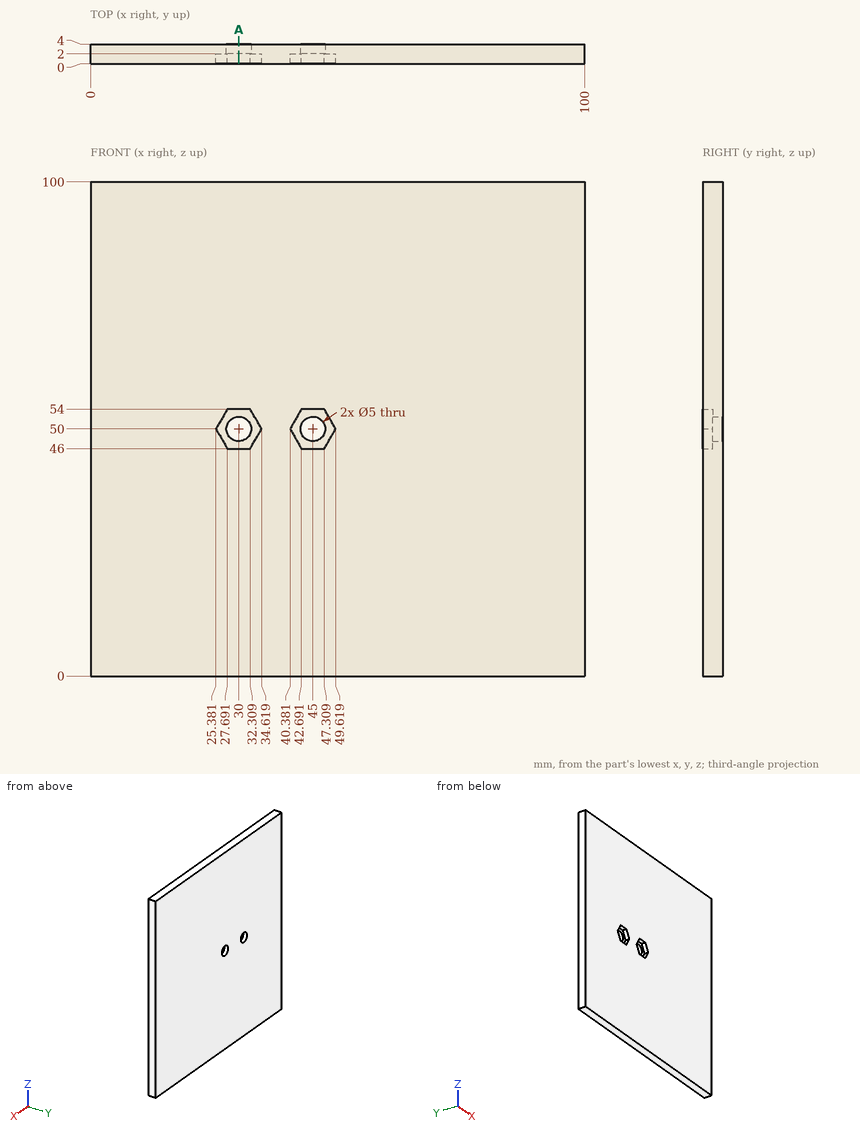
For this review, use the dimensioned drawing (mm, ordinates from the lowest corner) and the shaded views. Give positions to 0.01 mm unless a question says otherwise; leave off trailing zeros. Order: outer loops, then holes, each group sorted by start corner. A loop starts at its lowest first (then second) coordinate and runs counter-clockwise, first axis right, second up.
1. To check wall thickness, follow L1, parallel to X at y = 3.55, z = 50; L2, parallel to Z at x = 30, y = 2.7; L3, parallel to Z at x = 48.5, y = 0.75 (1 decimal). State the ranges of each line that lie inside material, in increasing order.
Solution:
L1: x = 0 to 27.5, 32.5 to 42.5, 47.5 to 100
L2: z = 0 to 47.5, 52.5 to 100
L3: z = 0 to 48.1, 51.9 to 100
2. Add section A-A, the plane x = 30. State the section outline as (y, z) points, then the cut area to 3 significant figures.
Solution:
outline: (0, 0) - (4, 0) - (4, 47.5) - (2, 47.5) - (2, 46) - (0, 46) - close; (0, 54) - (2, 54) - (2, 52.5) - (4, 52.5) - (4, 100) - (0, 100) - close
area: 374 mm2
3. For pin 1 Ø4.5 at (x, z) = (30, 50) entering from +Y; pin 2 Ø4 at (x, z) = (46, 50) entering from -Y, all flat-tipped, find the tip position at first contact; note any pin that passes through.
Solution:
pin 1: passes through
pin 2: stops at y = 2
